CAD build for the part. Positions are in the model's coordinates, mm. Face numbers are marked on the shaded views. A direction names the side the tool comes from. Coordinates: 2 decimals unless noted, no trailing zeros. Write each loop counter-clockwise with the first axis right and the second up, starting at its lowest first coordinate (ties: lowest second). Pieces come first, ordered by that corner, then holes. Notation, with made-up numbers: (-24, 72) - (5, 72) arc R6 cw to (5, 81) - close; hole circle Ø9 at (50.5, 31.5). An arc over 180 degrees is marked (long way). Answer in a Markdown table with one row per item. Add a question column.
Q1. Band-saw the part on A-A (y = 0). List the corners of the cut face in (x, z).
Q2. Two-plate mould, pull along Z, no slides. Class the marked faces 3, 4 and 5: +Z half, -Z half, draft (parallel to the pull), parting line (faces both ways), or undercut.
Q3. Pin check, flat tips, straight feed: pin 1 (12 mm diameter, centred on y = -26, z = 10, fed in from +X); pin 2 (3 mm diameter, centred on x = 5, z = -17, fed in from -Y); pin 3 (4 mm diameter, centred on y = 1, z = 0.5, fed in from -X). Stop position of each tip, or through.
Q4. 3-axis set-ups, long thin cutter, end or side, ignore diameter. For the marked faces 1 and 2: which of +Z, -Z, +X, -X, +Y, -Y reach the whole face in a straight line?
Q5. Band-saw the part on C-C (x = 5). List the corners of the cut face in (y, z), and give its area (3 significant figures).
Q6. Band-saw the part on D-D (x = 11.5). List the corners of the cut face in (y, z), and give its area (3 significant figures).
Q7. Drill centre lines: line 1 along Y through (x, z) = (4.95, 0); line 2 along X through (y, z) = (-18, -19.5); line 3 along X through (y, z) = (-1.5, -13.5). Where is each one in solid material? Low to high. Write a range as from..to.
```python
from build123d import *

# Parameters (mm, degrees)
SKETCH1_R           = 38.1
BOSS_EXTRUDE1_DEPTH = 10.16
SKETCH3_R           = 4.191
BOSS_EXTRUDE2_DEPTH = 2.54
SKETCH4_R           = 1.524
CUT_EXTRUDE1_DEPTH  = 13.7
SKETCH5_R           = 22.86
CUT_EXTRUDE2_DEPTH  = 3.81
SKETCH6_R           = 12.7
CUT_EXTRUDE3_DEPTH  = 2.54
SKETCH7_R           = 6.731
BOSS_EXTRUDE3_DEPTH = 3.81
SKETCH9_R           = 3.81
CUT_EXTRUDE4_DEPTH  = 3.81


with BuildPart() as part:
    # Sketch1 → Boss-Extrude1 (new body)
    with BuildSketch(Plane(origin=(0, 0, 0), x_dir=(0, 0, -1), z_dir=(1, 0, 0))):
        Circle(SKETCH1_R)
    extrude(amount=BOSS_EXTRUDE1_DEPTH)

    # Sketch3 → Boss-Extrude2 (add)
    with BuildSketch(Plane(origin=(10.16, 0, 0), x_dir=(0, 0, -1), z_dir=(1, 0, 0))):
        Circle(SKETCH3_R)
    extrude(amount=BOSS_EXTRUDE2_DEPTH)

    # Sketch4 → Cut-Extrude1 (cut, through all)
    with BuildSketch(Plane(origin=(12.7, 0, 0), x_dir=(0, 0, -1), z_dir=(1, 0, 0))):
        Circle(SKETCH4_R)
    extrude(amount=-CUT_EXTRUDE1_DEPTH, mode=Mode.SUBTRACT)

    # Sketch5 → Cut-Extrude2 (cut)
    with BuildSketch(Plane.ZY):
        Circle(SKETCH5_R)
    extrude(amount=-CUT_EXTRUDE2_DEPTH, mode=Mode.SUBTRACT)

    # Sketch6 → Cut-Extrude3 (cut)
    with BuildSketch(Plane.ZY.offset(-3.81)):
        Circle(SKETCH6_R)
    extrude(amount=-CUT_EXTRUDE3_DEPTH, mode=Mode.SUBTRACT)

    # Sketch7 → Boss-Extrude3 (add)
    with BuildSketch(Plane.ZY.offset(-6.35)):
        Circle(SKETCH7_R)
    extrude(amount=BOSS_EXTRUDE3_DEPTH)

    # Sketch9 → Cut-Extrude4 (cut)
    with BuildSketch(Plane.ZY.offset(-2.54)):
        Circle(SKETCH9_R)
    extrude(amount=-CUT_EXTRUDE4_DEPTH, mode=Mode.SUBTRACT)


solid = part.part
```
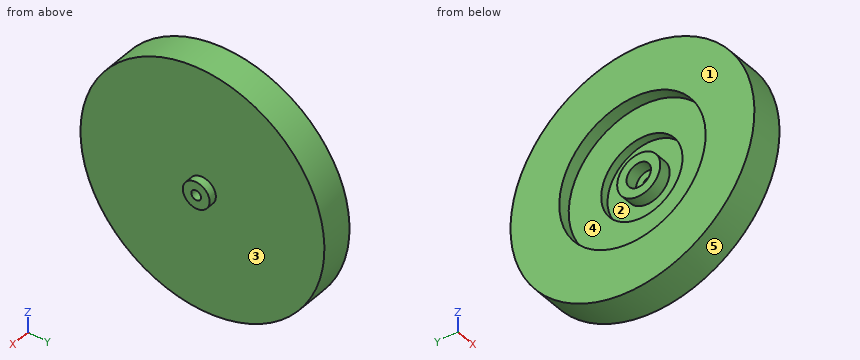
Checked values:
| question | item | result |
|---|---|---|
| 1 | outline | (0, -38.1) - (10.16, -38.1) - (10.16, -4.19) - (12.7, -4.19) - (12.7, -1.52) - (6.35, -1.52) - (6.35, -3.81) - (2.54, -3.81) - (2.54, -6.73) - (6.35, -6.73) - (6.35, -12.7) - (3.81, -12.7) - (3.81, -22.86) - (0, -22.86) - close; (0, 22.86) - (3.81, 22.86) - (3.81, 12.7) - (6.35, 12.7) - (6.35, 6.73) - (2.54, 6.73) - (2.54, 3.81) - (6.35, 3.81) - (6.35, 1.52) - (12.7, 1.52) - (12.7, 4.19) - (10.16, 4.19) - (10.16, 38.1) - (0, 38.1) - close |
| 2 | face 3 | draft |
| 2 | face 4 | undercut |
| 2 | face 5 | parting line |
| 3 | pin 1 | stops at x = 10.16 |
| 3 | pin 2 | stops at y = -34.8 |
| 3 | pin 3 | stops at x = 6.35 |
| 4 | face 1 | +Z, -Z, -X, +Y, -Y |
| 4 | face 2 | -X |
| 5 | outline | circle Ø76.2 at (0, 0); circle Ø13.46 at (0, 0); hole circle Ø25.4 at (0, 0); hole circle Ø7.62 at (0, 0) |
| 5 | area | 4,150 mm² |
| 6 | outline | circle Ø8.38 at (0, 0); hole circle Ø3.05 at (0, 0) |
| 6 | area | 47.9 mm² |
| 7 | line 1 | y = -38.1..-12.7, -6.73..-3.81, 3.81..6.73, 12.7..38.1 |
| 7 | line 2 | x = 0..10.16 |
| 7 | line 3 | x = 3.81..10.16 |
